Geometry check sheet. Reference: the model listing, model coordinates, mm. A direction names the side the tool comes from. Give positions to 0.01 mm unless a question says otherwise; leave off trailing zeros. Write each loop counter-clockwise with the first axis right and the second up, starting at its lowest first coordinate (ties: lowest second). Pieces come first, ordered by that corner, then holes. Notation, with made-up numbers: (-10, 14) - (39, 14) arc R29 cw to (39, 45) - close; hole circle Ø9 at (-22, 74). An arc over 180 degrees is marked (long way). Write item = value, one per line. Start each with the question number.
(1) Section check B-B, the plane y = 17. Enter the section's corners in (x, z), plus the area to 3 significant figures.
(2) Access from +Z, -Z, +X, -X, +Y, -Y to the whole of each face (thin tool, end or side, straight path). Record for faces 4 (the cylindrical face through (-10.874, 12.902, 0.887)), 5 (the flat face through (-8, -3, 0.875)).
(3) Draft check along X on faces 1 (the flat face through (-22.334, -3.206, 0.887)), 2 (the cylindrical face through (-10.874, -12.847, 0.887)), 3 (the flat face through (-5.8, -2.8, 0)). Enter one of: pulls with the +X half, pulls with the -X half, needs draft (parallel to the pull), parting line crosses it, or undercut.
(4) Section check A-A, the plane x = -1. Enter the section's corners in (y, z), plus the area to 3 significant figures.
(5) Thickness scan on L1, parallel to X at y = 14, z = 1.5; L2, parallel to Z at x = -10, y = 14; L3, parallel to Y at x = -10, z = -1.6. Record the ranges inside material, lowest first.
(6) Depth check by flat-ended pin: pin 1 Ø1.8 at (x, y) = (-9.5, 1.5) entering from -Z; pin 2 Ø3 at (x, y) = (-10.25, 0) entering from +Z (3 decimals). Enter the tip coordinate at first touch or a pass-through.
```python
from build123d import *

# Parameters (mm, degrees)
SKETCH1_R           = 4.5000037
BOSS_EXTRUDE1_DEPTH = 3.75000012
BOSS_EXTRUDE2_START = 1.750000056
SKETCH2_R           = 4.5000037
SKETCH2_R_2         = 3.499999998
SKETCH2_R_3         = 1.25000004
BOSS_EXTRUDE2_DEPTH = 1.750000056
SKETCH4_R           = 2.75000466
SKETCH4_R_2         = 1.25000004
CUT_EXTRUDE1_DEPTH  = 0.875000028
SKETCH6_R           = 4.5000037
SKETCH6_R_2         = 3.5000057
CUT_EXTRUDE2_DEPTH  = 0.875000028
SKETCH10_R          = 0.62500002
SKETCH10_R_2        = 4.5000037
BOSS_EXTRUDE4_DEPTH = 1.750000056
CHAMFER2_SIZE       = 1.00000054
CHAMFER2_SIZE2      = 0.577350581
SKETCH32_R          = 1.4605
CUT_EXTRUDE8_DEPTH  = 36.768264294


with BuildPart() as part:
    # Sketch1 → Boss-Extrude1 (new body)
    with BuildSketch(Plane.XY):
        with Locations((-10.24995918, 0)):
            Circle(SKETCH1_R)
        Polygon((-10.24995918, 2.999994), (-10.594624819, 2.728309468), (-10.996027349, 2.905743672), (-11.262299488, 2.55687975), (-11.695217312, 2.628914782), (-11.866365092, 2.224791874), (-12.303596391, 2.186901508), (-12.368865968, 1.752912142), (-12.782937891, 1.60747717), (-12.738228138, 1.170890494), (-13.103123023, 0.927049129), (-12.951243218, 0.515297489), (-13.244033377, 0.188371182), (-12.994526687, -0.172673551), (-13.196815038, -0.562142819), (-12.865358886, -0.849794878), (-12.964434908, -1.27733532), (-12.571855902, -1.473520467), (-12.561494285, -1.912268145), (-12.132459609, -2.004659346), (-12.01331141, -2.427046129), (-11.574778889, -2.409838105), (-11.354330629, -2.789323879), (-10.933854876, -2.663597874), (-10.625958129, -2.976338151), (-10.24995918, -2.749993992), (-9.873960231, -2.976338151), (-9.566063484, -2.663597874), (-9.145587731, -2.789323879), (-8.925139471, -2.409838105), (-8.48660695, -2.427046129), (-8.367458751, -2.004659346), (-7.938424075, -1.912268145), (-7.928062458, -1.473520467), (-7.535483452, -1.27733532), (-7.634559474, -0.849794878), (-7.303103322, -0.562142819), (-7.505391673, -0.172673551), (-7.255884983, 0.188371182), (-7.548675142, 0.515297489), (-7.396795337, 0.927049129), (-7.761690222, 1.170890494), (-7.716980469, 1.60747717), (-8.131052392, 1.752912142), (-8.196321969, 2.186901508), (-8.633553268, 2.224791874), (-8.804701048, 2.628914782), (-9.237618872, 2.55687975), (-9.503891011, 2.905743672), (-9.905293541, 2.728309468), align=None, mode=Mode.SUBTRACT)
    extrude(amount=-BOSS_EXTRUDE1_DEPTH)

    # Sketch2 → Boss-Extrude2 (add)
    # profile 1 of 2: a face of its own
    with BuildSketch(Plane.XY.offset(BOSS_EXTRUDE2_START)):
        with Locations((-10.24995918, 0)):
            Circle(SKETCH2_R)
        with Locations((-10.24995918, 0)):
            Circle(SKETCH2_R_2, mode=Mode.SUBTRACT)
    # profile 2 of 2: a face of its own
    with BuildSketch(Plane.XY.offset(BOSS_EXTRUDE2_START)):
        with Locations((-10.24995918, 0)):
            Circle(SKETCH2_R_2)
        with Locations((-10.24995918, 0)):
            Circle(SKETCH2_R_3, mode=Mode.SUBTRACT)
    extrude(amount=-BOSS_EXTRUDE2_DEPTH)

    # Sketch4 → Cut-Extrude1 (cut)
    with BuildSketch(Plane.XY.offset(1.750000056)):
        with Locations((-10.24995918, 0)):
            Circle(SKETCH4_R)
        with Locations((-10.24995918, 0)):
            Circle(SKETCH4_R_2, mode=Mode.SUBTRACT)
    extrude(amount=-CUT_EXTRUDE1_DEPTH, mode=Mode.SUBTRACT)

    # Sketch6 → Cut-Extrude2 (cut)
    with BuildSketch(Plane.XY.offset(1.750000056)):
        with Locations((-10.24995918, 0)):
            Circle(SKETCH6_R)
        with Locations((-10.24995918, 0)):
            Circle(SKETCH6_R_2, mode=Mode.SUBTRACT)
    extrude(amount=-CUT_EXTRUDE2_DEPTH, mode=Mode.SUBTRACT)

    # Sketch10 → Boss-Extrude4 (add)
    with BuildSketch(Plane.XY.offset(1.750000056)):
        with BuildLine():
            Line((-8.086927824, 17.701557226), (-6.029886341, 6.622035833))
            ThreePointArc((-6.029886341, 6.622035833), (-5.20161423, 5.04834495), (-3.627923347, 4.220072839))
            Line((-3.627923347, 4.220072839), (7.451598046, 2.163031356))
            ThreePointArc((7.451598046, 2.163031356), (9.25000182, 0), (7.451598046, -2.163031356))
            Line((7.451598046, -2.163031356), (-3.627923347, -4.220072839))
            ThreePointArc((-3.627923347, -4.220072839), (-5.20161423, -5.04834495), (-6.029886341, -6.622035833))
            Line((-6.029886341, -6.622035833), (-8.086927824, -17.701557226))
            ThreePointArc((-8.086927824, -17.701557226), (-10.24995918, -19.499961), (-12.412990536, -17.701557226))
            Line((-12.412990536, -17.701557226), (-14.470032019, -6.622035833))
            ThreePointArc((-14.470032019, -6.622035833), (-15.29830413, -5.04834495), (-16.871995013, -4.220072839))
            Line((-16.871995013, -4.220072839), (-27.951516406, -2.163031356))
            ThreePointArc((-27.951516406, -2.163031356), (-29.74992018, 0), (-27.951516406, 2.163031356))
            Line((-27.951516406, 2.163031356), (-16.871995013, 4.220072839))
            ThreePointArc((-16.871995013, 4.220072839), (-15.29830413, 5.04834495), (-14.470032019, 6.622035833))
            Line((-14.470032019, 6.622035833), (-12.412990536, 17.701557226))
            ThreePointArc((-12.412990536, 17.701557226), (-10.24995918, 19.499961), (-8.086927824, 17.701557226))
        make_face()
        with Locations((-10.24995918, 15.87496698)):
            Circle(SKETCH10_R, mode=Mode.SUBTRACT)
        with Locations((-10.24995918, 12.87497298)):
            Circle(SKETCH10_R, mode=Mode.SUBTRACT)
        with Locations((-10.24995918, 9.87497898)):
            Circle(SKETCH10_R, mode=Mode.SUBTRACT)
        with Locations((-10.24995918, 6.87498498)):
            Circle(SKETCH10_R, mode=Mode.SUBTRACT)
        with Locations((5.6250078, 0)):
            Circle(SKETCH10_R, mode=Mode.SUBTRACT)
        with Locations((2.6250138, 0)):
            Circle(SKETCH10_R, mode=Mode.SUBTRACT)
        with Locations((-0.3749802, 0)):
            Circle(SKETCH10_R, mode=Mode.SUBTRACT)
        with Locations((-3.3749742, 0)):
            Circle(SKETCH10_R, mode=Mode.SUBTRACT)
        with Locations((-10.24995918, -15.87496698)):
            Circle(SKETCH10_R, mode=Mode.SUBTRACT)
        with Locations((-10.24995918, -12.87497298)):
            Circle(SKETCH10_R, mode=Mode.SUBTRACT)
        with Locations((-10.24995918, -9.87497898)):
            Circle(SKETCH10_R, mode=Mode.SUBTRACT)
        with Locations((-10.24995918, -6.87498498)):
            Circle(SKETCH10_R, mode=Mode.SUBTRACT)
        with Locations((-26.12492616, 0)):
            Circle(SKETCH10_R, mode=Mode.SUBTRACT)
        with Locations((-23.12493216, 0)):
            Circle(SKETCH10_R, mode=Mode.SUBTRACT)
        with Locations((-20.12493816, 0)):
            Circle(SKETCH10_R, mode=Mode.SUBTRACT)
        with Locations((-17.12494416, 0)):
            Circle(SKETCH10_R, mode=Mode.SUBTRACT)
        with Locations((-10.24995918, 0)):
            Circle(SKETCH10_R_2, mode=Mode.SUBTRACT)
    extrude(amount=-BOSS_EXTRUDE4_DEPTH)

    # Chamfer2
    chamfer2_edges = [part.edges().sort_by_distance(p)[0] for p in [
        (-14.74996288, 0, 0),
    ]]
    chamfer2_side = [part.faces().sort_by_distance(p)[0] for p in [
        (-14.74996288, 0, -1.87500006),
    ]]
    chamfer(chamfer2_edges, length=CHAMFER2_SIZE, length2=CHAMFER2_SIZE2, reference=chamfer2_side[0])

    # Sketch32 → Cut-Extrude8 (cut, through all)
    with BuildSketch(Plane(origin=(0, 0, 0), x_dir=(-1, 0, 0), z_dir=(0, 0, -1))):
        with Locations((20.12493816, 0)):
            Circle(SKETCH32_R)
        with Locations((10.24995918, -9.87497898)):
            Circle(SKETCH32_R)
        with Locations((0.3749802, 0)):
            Circle(SKETCH32_R)
        with Locations((10.24995918, 9.87497898)):
            Circle(SKETCH32_R)
    extrude(amount=-CUT_EXTRUDE8_DEPTH, mode=Mode.SUBTRACT)


solid = part.part
```
Model answer:
q1.outline = (-12.54, 0) - (-7.96, 0) - (-7.96, 1.75) - (-12.54, 1.75) - close
q1.area = 8.03 mm²
q2.face_4 = +Z, -Z
q2.face_5 = +Z
q3.face_1 = pulls with the -X half
q3.face_2 = undercut
q3.face_3 = needs draft
q4.outline = (-3.73, 0) - (-1.32, 0) - (-1.32, 1.75) - (-3.73, 1.75) - close; (1.32, 0) - (3.73, 0) - (3.73, 1.75) - (1.32, 1.75) - close
q4.area = 8.44 mm²
q5.L1 = -13.1 to -7.4
q5.L2 = 0 to 1.75
q5.L3 = -4.49 to -2.9, 2.8 to 4.49
q6.pin_1 = 0
q6.pin_2 = 0.875
